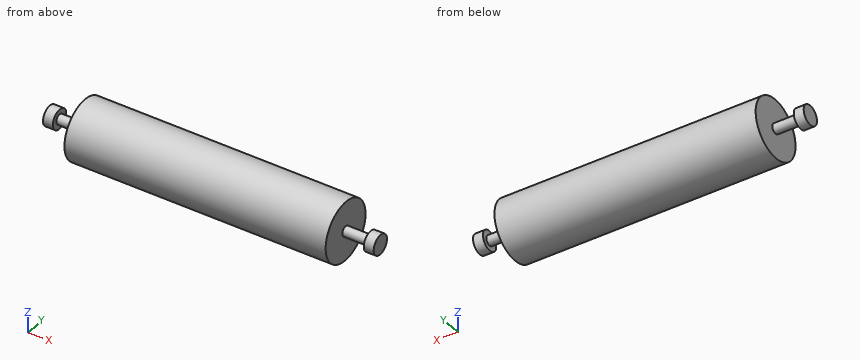
```python
from build123d import *

# Parameters (mm, degrees)
BOSS_EXTRUDE1_DEPTH      = 167.005
BOSS_EXTRUDE1_DEPTH_BACK = 167.005
SKETCH1_R                = 38.1
SKETCH2_R                = 6.35
BOSS_EXTRUDE2_DEPTH      = 31.75
SKETCH3_R                = 12.7
BOSS_EXTRUDE3_DEPTH      = 12.7


with BuildPart() as part:
    # Sketch1 → Boss-Extrude1 (new, two sides: drawn at the far end of the back side and taken through both)
    with BuildSketch(Plane(origin=(0, 0, 0), x_dir=(0, 0, -1), z_dir=(1, 0, 0)).offset(-BOSS_EXTRUDE1_DEPTH_BACK)):
        Circle(SKETCH1_R)
    extrude(amount=BOSS_EXTRUDE1_DEPTH + BOSS_EXTRUDE1_DEPTH_BACK)

    # Sketch2 → Boss-Extrude2 (add)
    with BuildSketch(Plane.ZY.offset(167.005)):
        Circle(SKETCH2_R)
    boss_extrude2 = extrude(amount=BOSS_EXTRUDE2_DEPTH)

    # Sketch3 → Boss-Extrude3 (add)
    with BuildSketch(Plane.ZY.offset(198.755)):
        Circle(SKETCH3_R)
    boss_extrude3 = extrude(amount=BOSS_EXTRUDE3_DEPTH)

    # Mirror1: Boss-Extrude2, Boss-Extrude3 across plane
    add(boss_extrude2.mirror(Plane(origin=(0, 0, 0), x_dir=(0, 0, 1), z_dir=(1, 0, 0))))
    add(boss_extrude3.mirror(Plane(origin=(0, 0, 0), x_dir=(0, 0, 1), z_dir=(1, 0, 0))))


solid = part.part
```
Verification items for the finished model (mm, model axes). Give positions to 0.01 mm unless a question says otherwise; leave off trailing zeros. Order: outer loops, then holes, each group sorted by start corner. A loop starts at its lowest first (then second) coordinate and runs counter-clockwise, first axis right, second up. Notation, with made-up numbers: M -16.5,-27 L 34.5,-27 A20 ccw 34.5,-7 Z; hole C -4,5 d9. An arc over 180 degrees is marked long. Return JSON: item names as keys, results as strings. Group by question number.
1) Scan lines: line 1 (X direction, y = -7.5, z = -2) (3 decimals); line 2 (X direction, y = 7, z = 32) (3 decimals); line 3 (Z direction, x = -115.5, y = -0.5). Record each from-to range of solid material in increasing order.
2) Section check A-A on y = 0. Record the cut outline in (x, z) (3 decimals).
3) Go/stop test with flat-tipped pins: pin 1 Ø2 at (y, z) = (-24.5, 11) entering from -X (3 decimals); pin 2 Ø8 at (x, y) = (139, -29.5) entering from -Z; pin 3 Ø5 at (x, z) = (107, -13.5) entering from -Y. Record where each tip stops, or that it passes through.
4) Section check C-C on x = 85. Record the cut outline in (y, z), and give its area (3 significant figures).
5) Section check D-D on z = 27. Record the cut outline in (x, y) (3 decimals).
Answer block:
{
 "1": {"line 1": "x = -211.455 to -198.755, -167.005 to 167.005, 198.755 to 211.455", "line 2": "x = -167.005 to 167.005", "line 3": "z = -38.1 to 38.1"},
 "2": {"outline": "M -211.455,-12.7 L -198.755,-12.7 L -198.755,-6.35 L -167.005,-6.35 L -167.005,-38.1 L 167.005,-38.1 L 167.005,-6.35 L 198.755,-6.35 L 198.755,-12.7 L 211.455,-12.7 L 211.455,12.7 L 198.755,12.7 L 198.755,6.35 L 167.005,6.35 L 167.005,38.1 L -167.005,38.1 L -167.005,6.35 L -198.755,6.35 L -198.755,12.7 L -211.455,12.7 Z"},
 "3": {"pin 1": "stops at x = -167.005", "pin 2": "stops at z = -28.31", "pin 3": "stops at y = -36.48"},
 "4": {"outline": "C 0,0 d76.2", "area": "4,560 mm^2"},
 "5": {"outline": "M -167.005,-26.881 L 167.005,-26.881 L 167.005,26.881 L -167.005,26.881 Z"}
}
